```python
from build123d import *

# Parameters (mm, degrees)
SKETCH1_R           = 4
BOSS_EXTRUDE1_DEPTH = 10
CHAMFER1_SIZE       = 5


with BuildPart() as part:
    # Sketch1 → Boss-Extrude1 (new body)
    with BuildSketch(Plane.XY):
        Polygon((0, 150), (56.4, 150), (56.4, 100), (46.4, 100), (46.4, 50), (56.4, 50), (56.4, 0), (0, 0), (0, 50), (10, 50), (10, 100), (0, 100), align=None)
        with Locations((28.2, 75)):
            Circle(SKETCH1_R, mode=Mode.SUBTRACT)
    extrude(amount=BOSS_EXTRUDE1_DEPTH)

    # Chamfer1
    chamfer1_edges = [part.edges().sort_by_distance(p)[0] for p in [
        (24.2, 75, 0),
    ]]
    chamfer(chamfer1_edges, length=CHAMFER1_SIZE)


solid = part.part
```
For this review, take the finished solid that the model builds, in its own axes (mm). A direction names the side the tool comes from. Coordinates: 2 decimals unless noted, no trailing zeros. Loops run counter-clockwise (first coordinate to the right, second up) from the corner with the lowest first, then second, coordinate; pieces in that order, holes last. Notation, with made-up numbers: (58, 33.5) -> (111, 33.5) arc R21 ccw to (111, 67.5) -> close; hole circle Ø4 at (16.25, -13). An arc over 180 degrees is marked (long way). Return JSON: item names as keys, results as strings. Group by question number.
(1) For pin 1 Ø3 at (y, z) = (65.5, 6) entering from -X; pin 2 Ø5 at (y, z) = (70.5, 6) entering from +X; pin 3 Ø7 at (x, y) = (28.2, 75) entering from +Z, all flat-tipped, find the tip position at first contact; note any pin that passes through.
(2) Mouldability with a two-part tool opening along Y and no side actions: class faces 4 (the flat face through (28, 150, 5)), 5 (the flat face through (0, 25, 5)), 6 (the flat face through (46.4, 75, 5)) as pulls with the +Y half, pulls with the -Y half, needs draft (parallel to the pull), parting line crosses it, or undercut.
(3) To check wall thickness, follow L1, parallel to Y at x = 28.2, z = 6.3; L2, parallel to Y at x = 47, z = 2.75; L3, parallel to X at y = 50.5, z = 0.5. State the ranges of each line that lie inside material, in increasing order.
(4) Tool access review of faces 1 (the flat face through (51, 50, 5)), 2 (the flat face through (5, 100, 5)), 3 (the flat face through (56.4, 125, 5)): name each direction out of +Z, -Z, +X, -X, +Y, -Y from which nothing blocks a thin tool from reaching the whole face with its end or side.
(5) Consider section A-A, the plane x = 28.2. Give the boundary of the cut face in (y, z).
(6) Consider section D-D, the plane x = 6. Give the boundary of the cut face in (y, z).
(7) Consider section C-C, the plane z = 3.5. Give the boundary of the cut face in (x, y), plus the area to 3 significant figures.
(8) Consider section B-B, the plane y = 75. Give the boundary of the cut face in (x, z).
Results below:
{
 "1": {"pin 1": "stops at x = 10", "pin 2": "stops at x = 46.4", "pin 3": "passes through"},
 "2": {"face 4": "pulls with the +Y half", "face 5": "needs draft", "face 6": "undercut"},
 "3": {"L1": "y = 0 to 71, 79 to 150", "L2": "y = 0 to 50, 100 to 150", "L3": "x = 10 to 46.4"},
 "4": {"face 1": "+Z, -Z, +X", "face 2": "+Z, -Z, -X", "face 3": "+Z, -Z, +X, +Y, -Y"},
 "5": {"outline": "(0, 0) -> (66, 0) -> (71, 5) -> (71, 10) -> (0, 10) -> close; (79, 5) -> (84, 0) -> (150, 0) -> (150, 10) -> (79, 10) -> close"},
 "6": {"outline": "(0, 0) -> (50, 0) -> (50, 10) -> (0, 10) -> close; (100, 0) -> (150, 0) -> (150, 10) -> (100, 10) -> close"},
 "7": {"outline": "(0, 0) -> (56.4, 0) -> (56.4, 50) -> (46.4, 50) -> (46.4, 100) -> (56.4, 100) -> (56.4, 150) -> (0, 150) -> (0, 100) -> (10, 100) -> (10, 50) -> (0, 50) -> close; hole circle Ø11 at (28.2, 75)", "area": "7,360 mm2"},
 "8": {"outline": "(10, 0) -> (19.2, 0) -> (24.2, 5) -> (24.2, 10) -> (10, 10) -> close; (32.2, 5) -> (37.2, 0) -> (46.4, 0) -> (46.4, 10) -> (32.2, 10) -> close"}
}
